Autodesk Inventor part; units mm, degrees
ref_plane "YZ Plane" through (0, 0, 0) normal (1, 0, 0) x (0, 1, 0)
ref_plane "XZ Plane" through (0, 0, 0) normal (0, 1, 0) x (-1, 0, 0)
ref_plane "XY Plane" through (0, 0, 0) normal (0, 0, 1) x (1, 0, 0)
sketch "Sketch1" plane through (0, 0, 0) normal (1, 0, 0) x (0, 1, 0)
  arc A0 (-6.35, -25.4) -> (6.35, -25.4) centre (0, -25.4) ccw
  line L0 (-6.35, -19.05) -> (-15.875, -19.05)
  circle A1 centre (-15.875, -12.7) radius 2.1844
  arc A2 (-22.225, -12.7) -> (-15.875, -19.05) centre (-15.875, -12.7) ccw
  line L1 (-6.35, -25.4) -> (-6.35, -19.05)
  circle A3 centre (15.875, -12.7) radius 2.1844
  arc A4 (15.875, -19.05) -> (22.225, -12.7) centre (15.875, -12.7) ccw
  line L2 (15.875, -19.05) -> (6.35, -19.05)
  line L3 (6.35, -19.05) -> (6.35, -25.4)
  circle A5 centre (0, 0) radius 2.1844
  circle A6 centre (0, -25.4) radius 2.1844
  line L4 (0, 6.35) -> (6.35, 6.35)
  line L5 (0, 6.35) -> (-6.35, 6.35)
  line L6 (-15.875, 6.35) -> (15.875, 6.35)
  line L7 (22.225, 0) -> (22.225, -12.7)
  line L8 (-6.35, 6.35) -> (-15.875, 6.35)
  line L9 (-22.225, 0) -> (-22.225, -12.7)
  circle A7 centre (15.875, 0) radius 2.1844
  circle A8 centre (-15.875, 0) radius 2.1844
  arc A9 (-15.875, 6.35) -> (-22.225, 0) centre (-15.875, 0) ccw
  arc A10 (22.225, 0) -> (15.875, 6.35) centre (15.875, 0) ccw
  dimension "d22" = 4.3688
  dimension "d23" = 4.3688
  dimension "d25" = 4.3688
  dimension "d27" = 4.3688
  dimension "d28" = 6.35
extrude "Extrusion1" add sketch "Sketch1" along normal blind 1.5875
properties part number "polygusset"
Here's how the part is built. I have some questions about the finished solid (model axes, mm). A direction names the side the tool comes from. Give positions to 0.01 mm unless a question says otherwise; leave off trailing zeros. Order: outer loops, then holes, each group sorted by start corner. A loop starts at its lowest first (then second) coordinate and runs counter-clockwise, first axis right, second up. Notation, with made-up numbers: (-4, -20.75) -> (30, -20.75) arc R18 cw to (30, 8.25) -> close; hole circle Ø7 at (77.25, 22). An arc over 180 degrees is marked (long way). Use a Markdown table: item, result. Add a question column.
Item 1: Imagine slicing it at A-A on y = 0. Please give me the cut outline in (x, z), plus the area to 3 significant figures.
Item 2: If we mould it in two halves opening along Y, with no side actions, what happens to faces 4 (the face through (0.78, 14.14, -11.37)), 5 (the face through (1, -6.35, -22)), 6 (the face through (1, 11, -19.05))? For each: pulls with the +Y half, pulls with the -Y half, needs draft (parallel to the pull), parting line crosses it, or undercut.
Item 3: Imagine slicing it at D-D on z = -18. Please give me the cut outline in (x, y), plus the area to 3 significant figures.
Item 4: Will these pins go through, and if not, where does the flat tip stop? pin 1 (0.8 mm diameter, centred on x = 1, z = -23.5, fed in from -Y); pin 2 (4 mm diameter, centred on y = 15.875, z = 0, fed in from -X); pin 3 (0.8 mm diameter, centred on x = 1, z = -23.5, fed in from +Y).
Item 5: Imagine slicing it at C-C on y = -16.5. Please give me the cut outline in (x, z), plus the area to 3 significant figures.
Item 6: Imagine slicing it at B-B on x = 1.3. Please give me the cut outline in (y, z) (3 decimals).
Item 7: For faces 1 (the face through (1, -11, -19.05)), 2 (the face through (1, 6.35, -22)), 3 (the face through (0.783, -18.057, -0.096)), which set-ups out of +Z, -Z, +X, -X, +Y, -Y let a thin tool reach every point of the face, with its end or its side?
Item 8: I need wall thicknesses on line 1 (Y direction, x = 0.4, z = -14); line 2 (Y direction, x = 1.2, z = -23); line 3 (Y direction, x = 0.45, z = -13). Which ranges of each line are inside material? Lowest first, please.
Data:
| question | item | result |
|---|---|---|
| 1 | outline | (0, -31.75) -> (1.59, -31.75) -> (1.59, -27.58) -> (0, -27.58) -> close; (0, -23.22) -> (1.59, -23.22) -> (1.59, -2.18) -> (0, -2.18) -> close; (0, 2.18) -> (1.59, 2.18) -> (1.59, 6.35) -> (0, 6.35) -> close |
| 1 | area | 46.6 mm² |
| 2 | face 4 | undercut |
| 2 | face 5 | pulls with the -Y half |
| 2 | face 6 | needs draft |
| 3 | outline | (0, -19.37) -> (1.59, -19.37) -> (1.59, 19.37) -> (0, 19.37) -> close |
| 3 | area | 61.5 mm² |
| 4 | pin 1 | stops at y = -6.35 |
| 4 | pin 2 | passes through |
| 4 | pin 3 | stops at y = 6.35 |
| 5 | outline | (0, -19.02) -> (1.59, -19.02) -> (1.59, -14.79) -> (0, -14.79) -> close; (0, -10.61) -> (1.59, -10.61) -> (1.59, -2.09) -> (0, -2.09) -> close; (0, 2.09) -> (1.59, 2.09) -> (1.59, 6.32) -> (0, 6.32) -> close |
| 5 | area | 26.9 mm² |
| 6 | outline | (-22.225, -12.7) arc R6.35 ccw to (-15.875, -19.05) -> (-6.35, -19.05) -> (-6.35, -25.4) arc R6.35 ccw to (6.35, -25.4) -> (6.35, -19.05) -> (15.875, -19.05) arc R6.35 ccw to (22.225, -12.7) -> (22.225, 0) arc R6.35 ccw to (15.875, 6.35) -> (-15.875, 6.35) arc R6.35 ccw to (-22.225, 0) -> close; hole circle Ø4.369 at (-15.875, -12.7); hole circle Ø4.369 at (-15.875, 0); hole circle Ø4.369 at (0, -25.4); hole circle Ø4.369 at (0, 0); hole circle Ø4.369 at (15.875, -12.7); hole circle Ø4.369 at (15.875, 0) |
| 7 | face 1 | -Z, +X, -X, -Y |
| 7 | face 2 | -Z, +X, -X, +Y |
| 7 | face 3 | +X, -X |
| 8 | line 1 | y = -22.09 to -17.63, -14.12 to 14.12, 17.63 to 22.09 |
| 8 | line 2 | y = -6.35 to 6.35 |
| 8 | line 3 | y = -22.22 to -18.04, -13.71 to 13.71, 18.04 to 22.22 |
